```python
from build123d import *

# Parameters (mm, degrees)
F0_W      = 14.75
F0_H      = 6
F0_R      = 1
F1_DEPTH  = 2
F2_W      = 2
F2_H      = 6
F3_DEPTH  = 14.75
F4_R      = 1
F5_DEPTH  = 25
F6_W      = 2
F6_H      = 6
F7_DEPTH  = 15
F8_R      = 1
F9_DEPTH  = 25
F10_W     = 2
F10_H     = 6
F11_DEPTH = 9.5
F12_W     = 6
F12_H     = 2
F13_DEPTH = 7
F14_R     = 1
F15_DEPTH = 25


with BuildPart() as f1:
    # F0 (on Front) → F1 (new body)
    with BuildSketch(Plane.XZ):
        with Locations((7.375, 3)):
            Rectangle(F0_W, F0_H)
        with Locations((11.75, 3)):
            Circle(F0_R, mode=Mode.SUBTRACT)
    extrude(amount=F1_DEPTH)

    # F2 (on face) → F3 (join)
    with BuildSketch(Plane.XZ.offset(2)):
        with Locations((1, 3)):
            Rectangle(F2_W, F2_H)
    extrude(amount=F3_DEPTH)

    # F4 (on face) → F5 (cut)
    with BuildSketch(Plane.YZ.offset(2)):
        with Locations((-13.75, 3)):
            Circle(F4_R)
    extrude(amount=-F5_DEPTH, mode=Mode.SUBTRACT)

    # F6 (on face) → F7 (join)
    with BuildSketch(Plane.XZ.offset(16.75)):
        with Locations((1, 3)):
            Rectangle(F6_W, F6_H)
    extrude(amount=F7_DEPTH)

    # F8 (on face) → F9 (cut)
    with BuildSketch(Plane.YZ.offset(2)):
        with Locations((-21.25, 3)):
            Circle(F8_R)
    extrude(amount=-F9_DEPTH, mode=Mode.SUBTRACT)

    # F10 (on face) → F11 (join)
    with BuildSketch(Plane.XY.offset(6)):
        with Locations((1, -28.75)):
            Rectangle(F10_W, F10_H)
    extrude(amount=F11_DEPTH)

    # F12 (on face) → F13 (join)
    with BuildSketch(Plane.YZ.offset(2)):
        with Locations((-28.75, 14.5)):
            Rectangle(F12_W, F12_H)
    extrude(amount=F13_DEPTH)

    # F14 (on face) → F15 (cut)
    with BuildSketch(Plane.XY.offset(15.5)):
        with Locations((6, -28.75)):
            Circle(F14_R)
    extrude(amount=-F15_DEPTH, mode=Mode.SUBTRACT)


solid = f1.part
```
Work out the finished part from the listing and answer in its coordinate system (mm). A direction names the side the tool comes from. Round coordinates to 2 decimals unless told otherwise and drop trailing zeros. Loops run counter-clockwise (first coordinate to the right, second up) from the corner with the lowest first, then second, coordinate; pieces in that order, holes last. Notation, with made-up numbers: (41, -20.5) -> (51, -20.5) arc R29 cw to (51, 3.5) -> close; hole circle Ø3 at (16, -16.5). An arc over 180 degrees is marked (long way). Write each question's results on one line, items separated by ' | '. Start each with the question number.
1. A tool of negligible diameter and unlimited length cuts with its end or side. For faces 1 (the face through (4.7, -28.8, 13.5)), 2 (the face through (1, -25.75, 13)), 3 (the face through (8, -2, 3)), from which of +Z, -Z, +X, -X, +Y, -Y can it reach the whole face along a straight path? Write none if from no direction.
2. Find the intervals of material crossed by probe 1 along Z at (x, y) = (11.75, -1.1); probe 2 along Z at (x, y) = (4, -30); probe 3 along Y at (x, z) = (6, 14.4), in increasing order. Write a range as from..to.
3. Section C-C (x = 6) is taken. Determine the outline of the cut face in (y, z), plus the area to 3 significant figures.
4. Section D-D (y = -21.25) is taken. Determine the outline of the cut face in (x, z).
5. For a pull along X with two mould halves and no side action, classify faces 4 (the face through (0, -20, 4)), 5 (the face through (1, -12, 0)), 6 (the face through (10.75, -0.99, 3.04)), 7 (the face through (5.87, -27.76, 14.51)) as +X half, -X half, draft (parallel to the pull), parting line (faces both ways), or undercut.
6. Section A-A (y = -28.75) is taken. Determine the outline of the cut face in (x, z).
7. Given pin 1 Ø5 at (x, y) = (6.5, -27.5) entering from -Z; pin 2 Ø1.6 at (y, z) = (-30, 14) entering from +X; pin 3 Ø1.8 at (x, y) = (6, -28.75) entering from +Z; pin 4 Ø8 at (x, z) = (3.5, 14) entering from +Y, each flat-ended and moving along its own axis, determine where each tip first touches the part or whether it passes through.
8. Section B-B (x = 11.75) is taken. Determine the outline of the cut face in (y, z), plus the area to 3 significant figures.
Evaluation:
1) face 1: -Z, +X, +Y, -Y | face 2: +Z, +X, -X, +Y | face 3: +Z, -Z, +X, -Y
2) probe 1: z = 0..2, 4..6 | probe 2: z = 13.5..15.5 | probe 3: y = -31.75..-29.75, -27.75..-25.75
3) outline: (-31.75, 13.5) -> (-29.75, 13.5) -> (-29.75, 15.5) -> (-31.75, 15.5) -> close; (-27.75, 13.5) -> (-25.75, 13.5) -> (-25.75, 15.5) -> (-27.75, 15.5) -> close; (-2, 0) -> (0, 0) -> (0, 6) -> (-2, 6) -> close | area: 20.0 mm2
4) outline: (0, 0) -> (2, 0) -> (2, 2) -> (0, 2) -> close; (0, 4) -> (2, 4) -> (2, 6) -> (0, 6) -> close
5) face 4: -X half | face 5: draft | face 6: undercut | face 7: undercut
6) outline: (0, 0) -> (2, 0) -> (2, 13.5) -> (5, 13.5) -> (5, 15.5) -> (0, 15.5) -> close; (7, 13.5) -> (9, 13.5) -> (9, 15.5) -> (7, 15.5) -> close
7) pin 1: stops at z = 13.5 | pin 2: stops at x = 9 | pin 3: passes through | pin 4: stops at y = -25.75
8) outline: (-2, 0) -> (0, 0) -> (0, 2) -> (-2, 2) -> close; (-2, 4) -> (0, 4) -> (0, 6) -> (-2, 6) -> close | area: 8.00 mm2
